Source: CAD feature listing. Evaluate the final solid. Frame: model axes, mm. Give positions to 0.01 mm unless a question says otherwise; leave off trailing zeros. Order: outer loops, then holes, each group sorted by start corner. A loop starts at its lowest first (then second) coordinate and runs counter-clockwise, first axis right, second up.
from build123d import *

# Parameters (mm, degrees)
SKETCH1_W          = 25
SKETCH1_H          = 3
SKETCH2_R          = 17.75
CUT_EXTRUDE1_DEPTH = 3
CHAMFER1_SIZE      = 1


with BuildPart() as part:
    # Sketch1 → Revolve1 (revolve)
    with BuildSketch(Plane.XY):
        with Locations((12.5, 1.5)):
            Rectangle(SKETCH1_W, SKETCH1_H)
    revolve(axis=Axis((25, 3, 0), (0, -1, 0)))

    # Sketch2 → Cut-Extrude1 (cut)
    with BuildSketch(Plane(origin=(0, 3, 0), x_dir=(1, 0, 0), z_dir=(0, 1, 0))):
        with Locations((25, 0)):
            Circle(SKETCH2_R)
    extrude(amount=-CUT_EXTRUDE1_DEPTH, mode=Mode.SUBTRACT)

    # Chamfer1
    chamfer1_edges = [part.edges().sort_by_distance(p)[0] for p in [
        (50, 3, 0),
    ]]
    chamfer(chamfer1_edges, length=CHAMFER1_SIZE)


solid = part.part
1) Section query C-C on y = 1.1. Output: boundary loops of the cut face in (x, z), and give its area (3 significant figures).
Checks:
outline: circle Ø50 at (25, 0); hole circle Ø35.5 at (25, 0)
area: 974 mm2
2) Section query B-B on z = 0. Output: boundary loops of the cut face in (x, y).
Checks:
outline: (0, 0) - (7.25, 0) - (7.25, 3) - (1, 3) - (0, 2) - close; (42.75, 0) - (50, 0) - (50, 2) - (49, 3) - (42.75, 3) - close
3) Ray query, L1, parallel to Z at x = 25, y = 2; L2, parallel to X at y = 1.95, z = 0; L3, parallel to X at y = 0.25, z = 12.5. Return the intervals inside material, ascending.
Checks:
L1: z = -25 to -17.75, 17.75 to 25
L2: x = 0 to 7.25, 42.75 to 50
L3: x = 3.35 to 12.4, 37.6 to 46.65
4) Section query A-A on x = 25. Output: boundary loops of the cut face in (y, z).
Checks:
outline: (0, -25) - (2, -25) - (3, -24) - (3, -17.75) - (0, -17.75) - close; (0, 17.75) - (3, 17.75) - (3, 24) - (2, 25) - (0, 25) - close
5) First-contact query: pin 1 Ø12 at (x, z) = (22, 13.5) entering from +Y. Flat tip, straight axial feed; report the tip coordinate or a pass-through.
Checks:
pin 1: stops at y = 3
